Verification items for this drawing (mm, ordinates from the low corner). A direction names the side the tool comes from. Give positions to 0.01 mm unless a question says otherwise; leave off trailing zeros. Loops run counter-clockwise (first coordinate to the right, second up) from the corner with the lowest first, then second, coordinate; pieces in that order, holes last. Notation, with made-up numbers: M -31.5,-32.75 L -5.5,-32.75 A12 ccw -5.5,-22.75 Z; hole C 16.5,72 d3. An arc over 180 degrees is marked long. Use a Markdown table: item, result.
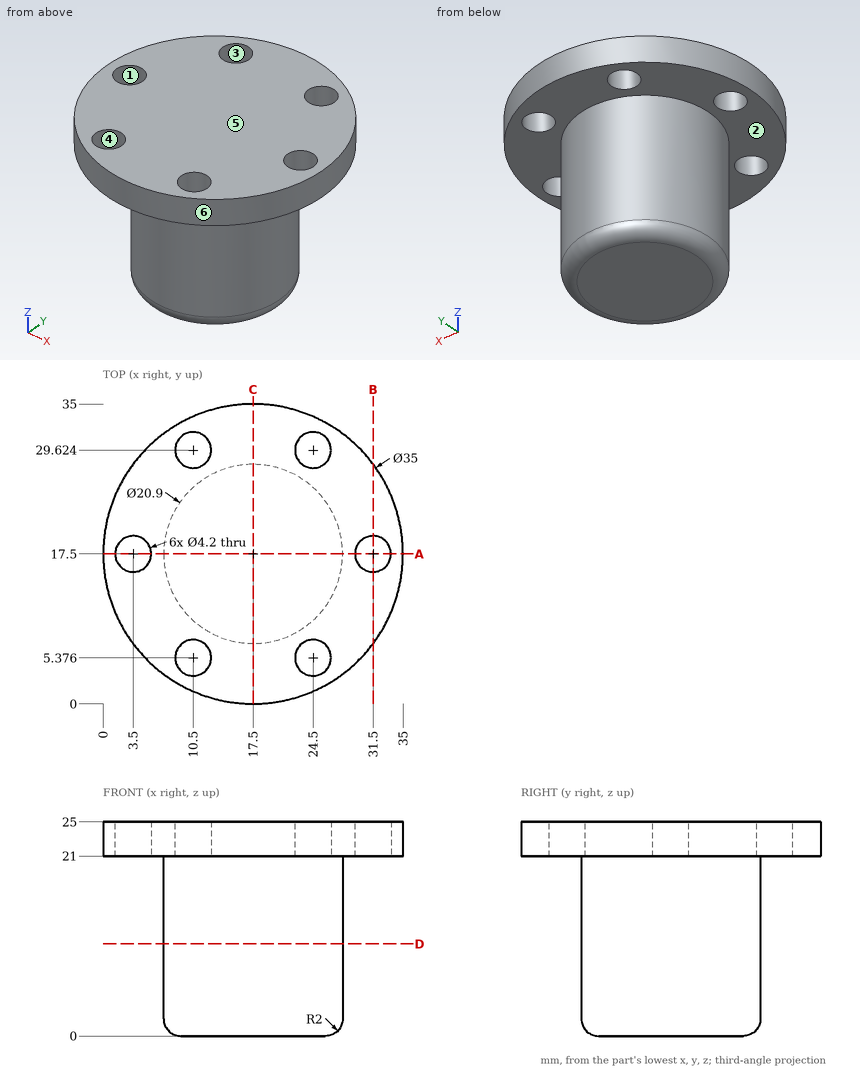
(1) Cross-section at D-D on z = 10.75. Record the cut outline in (x, y).
Results below:
| item | result |
|---|---|
| outline | C 17.5,17.5 d20.9 |
(2) Gauge pin test, flat ends, axial feed: P1, Ø1, axis at y = 18, z = 18.5, coming from the -X side; P2, Ø4, axis at x = 10.5, y = 29.62, coming from the -Z side; P3, Ø6.5, axis at x = 10.5, y = 5.38, coming from the -Z side; P4, Ø1.5, axis at y = 22, z = 8.5, coming from the +X side. Record the tip position at first contact, or that the pin passes through.
Results below:
| item | result |
|---|---|
| P1 | x = 7.05 |
| P2 | through |
| P3 | z = 21 |
| P4 | x = 27.25 |
(3) Draft check along Y on the marked faces 3, 4, 5 and 6. Enter one of: +Y half, -Y half, draft (parallel to the pull), parting line (faces both ways), or undercut.
Results below:
| item | result |
|---|---|
| face 3 | undercut |
| face 4 | undercut |
| face 5 | draft |
| face 6 | parting line |
(4) Set-up check for the marked faces 1 and 2: record each of +Z, -Z, +X, -X, +Y, -Y from which the full face is reachable in a straight line by a thin tool's end or side.
Results below:
| item | result |
|---|---|
| face 1 | +Z, -Z |
| face 2 | -Z |
(5) Cross-section at C-C on x = 17.5. Record the cut outline in (y, z), then the cut area to 3 significant figures.
Results below:
| item | result |
|---|---|
| outline | M 0,21 L 7.05,21 L 7.05,2 A2 ccw 9.05,0 L 25.95,0 A2 ccw 27.95,2 L 27.95,21 L 35,21 L 35,25 L 0,25 Z |
| area | 577 mm^2 |
(6) Cross-section at B-B on x = 31.5. Record the cut outline in (y, z), then the cut area to 3 significant figures.
Results below:
| item | result |
|---|---|
| outline | M 7,21 L 15.4,21 L 15.4,25 L 7,25 Z; M 19.6,21 L 28,21 L 28,25 L 19.6,25 Z |
| area | 67.2 mm^2 |
(7) Material ranges on line 1 (Y direction, x = 24.5, z = 21.85) (1 decimal); line 2 (Z direction, x = 32, y = 10.5); line 3 (Y direction, x = 31.5, z = 23.4), recorded low to high.
Results below:
| item | result |
|---|---|
| line 1 | 1.5 to 3.3, 7.5 to 27.5, 31.7 to 33.5 |
| line 2 | 21 to 25 |
| line 3 | 7 to 15.4, 19.6 to 28 |
(8) Cross-section at A-A on y = 17.5. Record the cut outline in (x, z).
Results below:
| item | result |
|---|---|
| outline | M 0,21 L 1.4,21 L 1.4,25 L 0,25 Z; M 5.6,21 L 7.05,21 L 7.05,2 A2 ccw 9.05,0 L 25.95,0 A2 ccw 27.95,2 L 27.95,21 L 29.4,21 L 29.4,25 L 5.6,25 Z; M 33.6,21 L 35,21 L 35,25 L 33.6,25 Z |
